from build123d import *

# Parameters (mm, degrees)
SKETCH1_R           = 3.96875
BOSS_EXTRUDE1_DEPTH = 16.5
SKETCH2_R           = 8.475
BOSS_EXTRUDE2_DEPTH = 1.4
CUT_EXTRUDE1_DEPTH  = 3


with BuildPart() as part:
    # Sketch1 → Boss-Extrude1 (new body)
    with BuildSketch(Plane(origin=(0, 0, 0), x_dir=(1, 0, 0), z_dir=(0, 1, 0))):
        Circle(SKETCH1_R)
    extrude(amount=BOSS_EXTRUDE1_DEPTH)

    # Sketch2 → Boss-Extrude2 (add)
    with BuildSketch(Plane(origin=(0, 16.5, 0), x_dir=(1, 0, 0), z_dir=(0, 1, 0))):
        Circle(SKETCH2_R)
    extrude(amount=BOSS_EXTRUDE2_DEPTH)

    # Sketch3 → Revolve2 (revolve)
    with BuildSketch(Plane.XY):
        with BuildLine():
            Line((-3.625, 20.4), (0, 20.4))
            Line((0, 20.4), (0, 17.9))
            Line((0, 17.9), (-6.625, 17.9))
            ThreePointArc((-6.625, 17.9), (-5.275236962, 19.330284354), (-3.625, 20.4))
        make_face()
    revolve(axis=Axis((0, 20.4, 0), (0, -1, 0)))

    # Sketch4 → Cut-Extrude1 (cut)
    with BuildSketch(Plane(origin=(0, 20.4, 0), x_dir=(1, 0, 0), z_dir=(0, 1, 0))):
        Polygon((-2.38125, 1.374815329), (-2.38125, -1.374815329), (0, -2.749630657), (2.38125, -1.374815329), (2.38125, 1.374815329), (0, 2.749630657), align=None)
    extrude(amount=-CUT_EXTRUDE1_DEPTH, mode=Mode.SUBTRACT)


solid = part.part
Read the model definition and answer for the solid it produces. Units are mm, in the model's axes. A direction names the side the tool comes from. Coordinates: 2 decimals unless noted, no trailing zeros. Loops run counter-clockwise (first coordinate to the right, second up) from the corner with the lowest first, then second, coordinate; pieces in that order, holes last.
Q1. Each of these flat-tipped pins is pushed along its axis until it touches: pin 1 Ø3 at (x, z) = (-6.5, -1.5) entering from +Y; pin 2 Ø3 at (x, y) = (-3, 2) entering from -Z; pin 3 Ø0.8 at (y, z) = (19.5, 0.5) entering from +X. Where does it stop, or does it pass through?
Q2. The part is cut by section D-D on z = -6.25. Write down the section's boundary in (x, y), and give its area (3 significant figures).
Q3. The part is cut by section A-A on z = 0. Write down the section's boundary in (x, y) (3 decimals), and give its area (3 significant figures).
Q4. The part is cut by section C-C on x = 2. Write down the section's boundary in (y, z).
Q5. Consider probe 1 along Y at (x, z) = (-0.25, -6.75); probe 2 along X at (y, z) = (12, 0); probe 3 along Z at (x, y) = (2, 19). Determine where each line is inside the solid, lowest interval first.
Q6. The part is cut by section B-B on y = 5.5. Write down the section's boundary in (x, z).
Q7. Which of the six approach directions +Z, -Z, +X, -X, +Y, -Y give full straight-line access (tool end or side, diameter ignored) to faces 4 (the face through (4, 17.9, 6)), 5 (the face through (2, 16.5, 4)), 6 (the face through (0.9, 20.4, -2.5))?
Q8. The mould has two halves that part along X. Classify faces 1 (the face through (0, 0, 0)), 2 (the face through (-6.246, 17.19, -5.728)), 3 (the face through (0, 17.4, 0)): +X half, -X half, draft (parallel to the pull), parting line (faces both ways), or undercut.
Results below:
1. pin 1: stops at y = 19.42
1. pin 2: stops at z = -3.67
1. pin 3: stops at x = 5.52
2. outline: (-5.72, 16.5) - (5.72, 16.5) - (5.72, 17.9) - (2.2, 17.9) arc R5.37 ccw to (-2.2, 17.9) - (-5.72, 17.9) - close
2. area: 17.4 mm2
3. outline: (-8.475, 16.5) - (-3.969, 16.5) - (-3.969, 0) - (3.969, 0) - (3.969, 16.5) - (8.475, 16.5) - (8.475, 17.9) - (6.625, 17.9) arc R8.24 ccw to (3.625, 20.4) - (2.381, 20.4) - (2.381, 17.4) - (-2.381, 17.4) - (-2.381, 20.4) - (-3.625, 20.4) arc R8.24 ccw to (-6.625, 17.9) - (-8.475, 17.9) - close
3. area: 167 mm2
4. outline: (0, -3.43) - (16.5, -3.43) - (16.5, -8.24) - (17.9, -8.24) - (17.9, -6.32) arc R7.99 ccw to (20.4, -3.02) - (20.4, -1.59) - (17.4, -1.59) - (17.4, 1.59) - (20.4, 1.59) - (20.4, 3.02) arc R7.99 ccw to (17.9, 6.32) - (17.9, 8.24) - (16.5, 8.24) - (16.5, 3.43) - (0, 3.43) - close
5. probe 1: y = 16.5 to 17.9
5. probe 2: x = -3.97 to 3.97
5. probe 3: z = -5.28 to -1.59, 1.59 to 5.28
6. outline: circle Ø7.94 at (0, 0)
7. face 4: +Y
7. face 5: -Y
7. face 6: +Z, -Z, +X, -X, +Y
8. face 1: draft
8. face 2: parting line
8. face 3: undercut
